```python
from build123d import *

# Parameters (mm, degrees)
BOSS_EXTRUDE1_DEPTH       = 36
SKETCH2_R                 = 11
BOSS_EXTRUDE2_DEPTH       = 2
SKETCH3_R                 = 2.5
BOSS_EXTRUDE3_DEPTH       = 21
M3X0_5_TAPPED_HOLE1_D     = 2.5
M3X0_5_TAPPED_HOLE1_DEPTH = 5
M3X0_5_TAPPED_HOLE1_TIP   = 0.751075774


with BuildPart() as part:
    # Sketch1 → Boss-Extrude1 (new body)
    with BuildSketch(Plane.XY):
        Polygon((-14.003805752, -17.6), (14.003805752, -17.6), (17.6, -14.003805752), (17.6, 14.003805752), (14.003805752, 17.6), (-14.003805752, 17.6), (-17.6, 14.003805752), (-17.6, -14.003805752), align=None)
    extrude(amount=-BOSS_EXTRUDE1_DEPTH)

    # Sketch2 → Boss-Extrude2 (add)
    with BuildSketch(Plane.XY):
        Circle(SKETCH2_R)
    extrude(amount=BOSS_EXTRUDE2_DEPTH)

    # Sketch3 → Boss-Extrude3 (add)
    with BuildSketch(Plane.XY):
        Circle(SKETCH3_R)
    extrude(amount=BOSS_EXTRUDE3_DEPTH)

    # M3x0.5 Tapped Hole1
    with Locations(Plane.XY):
        with Locations((-13, -13), (13, -13), (13, 13), (-13, 13)):
            Hole(M3X0_5_TAPPED_HOLE1_D / 2, depth=M3X0_5_TAPPED_HOLE1_DEPTH)
            with Locations((0, 0, -(M3X0_5_TAPPED_HOLE1_DEPTH + M3X0_5_TAPPED_HOLE1_TIP / 2))):  # 118° drill point
                Cone(0, M3X0_5_TAPPED_HOLE1_D / 2, M3X0_5_TAPPED_HOLE1_TIP, mode=Mode.SUBTRACT)


solid = part.part
```
Source: CAD feature listing. Evaluate the final solid. Frame: model axes, mm. A direction names the side the tool comes from. Round coordinates to 2 decimals unless told otherwise and drop trailing zeros. Loops run counter-clockwise (first coordinate to the right, second up) from the corner with the lowest first, then second, coordinate; pieces in that order, holes last. Notation, with made-up numbers: (-6, 70) - (18, 70) arc R13 cw to (18, 93) - close; hole circle Ø3 at (41.25, 59.25). An arc over 180 degrees is marked (long way). Use CSV: the item, a comma, the result in double quotes.
Q1. Pin query (flat end, axial travel): pin 1 Ø4 at (x, y) = (13, 13) entering from +Z; pin 2 Ø1 at (x, z) = (4.5, 13.5) entering from -Y; pin 3 Ø1 at (x, y) = (-4, 1) entering from +Z. Return the tip coordinate at first contact, or that it passes through.
Reported:
pin 1,"z = 0"
pin 2,"through"
pin 3,"z = 2"
Q2. Section query C-C, the plane y = -6. Output: boundary loops of the cut face in (x, z).
Reported:
outline,"(-17.6, -36) - (17.6, -36) - (17.6, 0) - (9.22, 0) - (9.22, 2) - (-9.22, 2) - (-9.22, 0) - (-17.6, 0) - close"
Q3. Ray query, line 1 along X through (y, z) = (-13, -1); line 2 along Z through (x, y) = (4.5, 14). Return the intervals inside material, ascending.
Reported:
line 1,"-17.6 to -14.25, -11.75 to 11.75, 14.25 to 17.6"
line 2,"-36 to 0"
Q4. Reachability of faces 1 (the flat face through (0, 17.6, -18)), 2 (the cylindrical face through (-12.84, -11.76, -2.54)) from +Z, -Z, +X, -X, +Y, -Y: full face, straight path, thin tool, end or side. Return the list, or none.
Reported:
face 1,"+Z, -Z, +X, -X, +Y"
face 2,"+Z"
Q5. Section query D-D, the plane x = 0. Output: boundary loops of the cut face in (y, z), then the cut area to 3 significant figures.
Reported:
outline,"(-17.6, -36) - (17.6, -36) - (17.6, 0) - (11, 0) - (11, 2) - (2.5, 2) - (2.5, 21) - (-2.5, 21) - (-2.5, 2) - (-11, 2) - (-11, 0) - (-17.6, 0) - close"
area,"1,410 mm^2"
Q6. Mould query, pull axis X, two halves, no side actions, for faces 3 (the conical face through (12.84, 13.15, -5.62)), 4 (the flat face through (-17.6, 0, -18)), 5 (the flat face through (17.6, 0, -18)). Classes: pulls with the +X half, pulls with the -X half, needs draft (parallel to the pull), parting line crosses it, or undercut.
Reported:
face 3,"undercut"
face 4,"pulls with the -X half"
face 5,"pulls with the +X half"
Q7. Section query A-A, the plane z = -2.5. Output: boundary loops of the cut face in (x, y), then the cut area to 3 significant figures.
Reported:
outline,"(-17.6, -14) - (-14, -17.6) - (14, -17.6) - (17.6, -14) - (17.6, 14) - (14, 17.6) - (-14, 17.6) - (-17.6, 14) - close; hole circle Ø2.5 at (-13, -13); hole circle Ø2.5 at (-13, 13); hole circle Ø2.5 at (13, -13); hole circle Ø2.5 at (13, 13)"
area,"1,190 mm^2"
Q8. Section query B-B, the plane z = -31. Output: boundary loops of the cut face in (x, y), then the cut area to 3 significant figures.
Reported:
outline,"(-17.6, -14) - (-14, -17.6) - (14, -17.6) - (17.6, -14) - (17.6, 14) - (14, 17.6) - (-14, 17.6) - (-17.6, 14) - close"
area,"1,210 mm^2"
